```python
from build123d import *

# Parameters (mm, degrees)
SKETCH6_R               = 6
BOSS_EXTRUDE4_DEPTH     = 10
SKETCH7_R               = 3
BOSS_EXTRUDE5_DEPTH     = 30
CHAMFER1_SIZE           = 0.3
CHAMFER2_SIZE           = 0.3
CUT_EXTRUDE4_DEPTH      = 43.190046219
CUT_EXTRUDE4_DEPTH_BACK = 43.190046219
SKETCH10_R              = 1.55
CUT_EXTRUDE5_DEPTH      = 41.890096728
CUT_EXTRUDE5_DEPTH_BACK = 41.890096728
SKETCH11_R              = 2.6
FILLET1_R               = 1


with BuildPart() as part:
    # Sketch6 → Boss-Extrude4 (new body)
    with BuildSketch(Plane(origin=(0, 0, 0), x_dir=(1, 0, 0), z_dir=(0, 1, 0))):
        with Locations(Location((0, 0, 0), (0, 0, 270))):
            Circle(SKETCH6_R)
    extrude(amount=BOSS_EXTRUDE4_DEPTH)

    # Sketch7 → Boss-Extrude5 (add)
    with BuildSketch(Plane(origin=(0, 10, 0), x_dir=(1, 0, 0), z_dir=(0, 1, 0))):
        with Locations(Location((0, 0, 0), (0, 0, 270))):
            Circle(SKETCH7_R)
    extrude(amount=BOSS_EXTRUDE5_DEPTH)

    # Chamfer1
    chamfer1_edges = [part.edges().sort_by_distance(p)[0] for p in [
        (0, 40, -3),
    ]]
    chamfer(chamfer1_edges, length=CHAMFER1_SIZE)

    # Chamfer2
    chamfer2_edges = [part.edges().sort_by_distance(p)[0] for p in [
        (0, 10, -6),
    ]]
    chamfer(chamfer2_edges, length=CHAMFER2_SIZE)

    # Sketch10 → Cut-Extrude4 (cut, two sides: drawn at the far end of the back side and taken through both)
    with BuildSketch(Plane.ZY.offset(6).offset(-CUT_EXTRUDE4_DEPTH_BACK)):
        with Locations((0, 4.567060469)):
            Circle(SKETCH10_R)
    extrude(amount=CUT_EXTRUDE4_DEPTH + CUT_EXTRUDE4_DEPTH_BACK, mode=Mode.SUBTRACT)

    # Sketch11 → Cut-Extrude5 (cut, two sides: drawn at the far end of the back side and taken through both)
    with BuildSketch(Plane(origin=(0, 40, 0), x_dir=(1, 0, 0), z_dir=(0, 1, 0)).offset(-CUT_EXTRUDE5_DEPTH_BACK)):
        with Locations(Location((0, 0, 0), (0, 0, 270))):
            Circle(SKETCH11_R)
    extrude(amount=CUT_EXTRUDE5_DEPTH + CUT_EXTRUDE5_DEPTH_BACK, mode=Mode.SUBTRACT)

    # Fillet1
    fillet1_edges = [part.edges().sort_by_distance(p)[0] for p in [
        (0, 10, -3),
    ]]
    fillet(fillet1_edges, radius=FILLET1_R)


solid = part.part
```
Could you check a few things on this model? Use its own coordinates, in mm. A direction names the side the tool comes from. Round coordinates to 2 decimals unless told otherwise and drop trailing zeros. Loops run counter-clockwise (first coordinate to the right, second up) from the corner with the lowest first, then second, coordinate; pieces in that order, holes last. Notation, with made-up numbers: (77, 9) - (82, 9) arc R24 cw to (82, 23) - close; hole circle Ø6 at (32.25, 49). An arc over 180 degrees is marked (long way). Answer in a Markdown table with one row per item. Add a question column.
(1) I need wall thicknesses on line 1 along X through (y, z) = (25.5, 0); line 2 along Y through (x, z) = (4.35, 0); line 3 along X through (y, z) = (10.5, 0). Which ranges of each line are inside material? Lowest first, please.
(2) If we section it at A-A (z = 0): Please give me the cut outline in (x, y), plus the area to 3 significant figures.
(3) For faces 1 (the face through (-4, 10, 2)), 2 (the face through (-5.323, 4.782, 2.769)), which set-ups out of +Z, -Z, +X, -X, +Y, -Y let a thin tool reach every point of the face, with its end or its side?
(4) If we mould it in two halves opening along Y, with no side actions, what happens to faces 3 (the face through (-4.02, 3.97, 1.43)), 4 (the face through (0.9, 25.15, 2.86)), 5 (the face through (-1, 0, 3)), 6 (the face through (4.074, 3.054, -0.336))? For each: pulls with the +Y half, pulls with the -Y half, needs draft (parallel to the pull), parting line crosses it, or undercut.
(5) I'm going to push flat-ended pins straight in: pin 1 (1.5 mm diameter, centred on x = 1, y = 25, fed in from +Z); pin 2 (5 mm diameter, centred on y = 12, z = -4.5, fed in from +X). Where does each tip first touch, or does it pass through?
(6) If we section it at B-B (x = 0): Please give me the cut outline in (y, z), plus the area to 3 significant figures.
(7) If we section it at C-C (y = 7.5): Please give me the cut outline in (x, z), plus the area to 3 significant figures.
(8) If we section it at D-D (y = 14.5): Please give me the cut outline in (x, z), plus the area to 3 significant figures.
Model answer:
| question | item | result |
|---|---|---|
| 1 | line 1 | x = -3 to -2.6, 2.6 to 3 |
| 1 | line 2 | y = 0 to 3.02, 6.12 to 10 |
| 1 | line 3 | x = -3.13 to -2.6, 2.6 to 3.13 |
| 2 | outline | (-6, 0) - (-2.6, 0) - (-2.6, 3.02) - (-6, 3.02) - close; (-6, 6.12) - (-2.6, 6.12) - (-2.6, 40) - (-2.7, 40) - (-3, 39.7) - (-3, 11) arc R1 cw to (-4, 10) - (-5.7, 10) - (-6, 9.7) - close; (2.6, 0) - (6, 0) - (6, 3.02) - (2.6, 3.02) - close; (2.6, 6.12) - (6, 6.12) - (6, 9.7) - (5.7, 10) - (4, 10) arc R1 cw to (3, 11) - (3, 39.7) - (2.7, 40) - (2.6, 40) - close |
| 2 | area | 71.2 mm² |
| 3 | face 1 | +Y |
| 3 | face 2 | +Y, -Y |
| 4 | face 3 | undercut |
| 4 | face 4 | needs draft |
| 4 | face 5 | pulls with the -Y half |
| 4 | face 6 | undercut |
| 5 | pin 1 | stops at z = 2.99 |
| 5 | pin 2 | stops at x = 4.88 |
| 6 | outline | (0, -6) - (9.7, -6) - (10, -5.7) - (10, -4) arc R1 cw to (11, -3) - (39.7, -3) - (40, -2.7) - (40, -2.6) - (0, -2.6) - close; (0, 2.6) - (40, 2.6) - (40, 2.7) - (39.7, 3) - (11, 3) arc R1 cw to (10, 4) - (10, 5.7) - (9.7, 6) - (0, 6) - close |
| 6 | area | 92.2 mm² |
| 7 | outline | circle Ø12 at (0, 0); hole circle Ø5.2 at (0, 0) |
| 7 | area | 91.9 mm² |
| 8 | outline | circle Ø6 at (0, 0); hole circle Ø5.2 at (0, 0) |
| 8 | area | 7.04 mm² |
